Model file for the job. Use its own axes, mm. Coordinates: 2 decimals unless noted, no trailing zeros. Order: outer loops, then holes, each group sorted by start corner. A loop starts at its lowest first (then second) coordinate and runs counter-clockwise, first axis right, second up. Notation, with made-up numbers: M 3.25,44 L 62.25,44 A19 cw 62.25,53 Z; hole C -37.75,-38.75 d6. An arc over 180 degrees is marked long. Return JSON: item names as keys, results as strings.
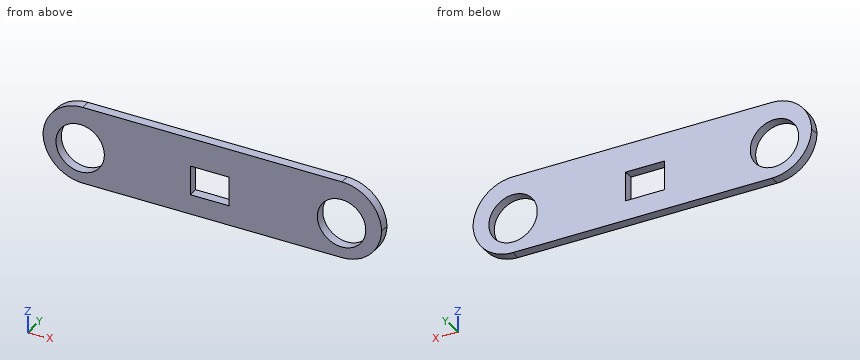
```python
from build123d import *

# Parameters (mm, degrees)
F0_R        = 31.75
F0_W        = 50.8
F0_H        = 38.4544562548
F1_DEPTH    = 12.7
F2_T1_DEPTH = 273.2826573419
F2_T3_DEPTH = 273.264091489
F2_T5_DEPTH = 273.3012245177


# Not quite as in the source:
# - a fillet or chamfer that OpenCascade refuses, or shapes differently, is made with other operations: its cross-section is extruded or revolved along the edge and cut away or added


with BuildPart() as f1:
    # F0 (on Front) → F1 (new body)
    with BuildSketch(Plane.XZ):
        Polygon((248.1590109615, 55.626), (-196.0797500385, 55.626), (-196.0869890385, -45.974), (248.1590109615, -45.974), align=None)
        with Locations((-147.3189890385, 0)):
            Circle(F0_R, mode=Mode.SUBTRACT)
        with Locations((22.6070109615, -0.7874006405)):
            Rectangle(F0_W, F0_H, mode=Mode.SUBTRACT)
        with Locations((195.5810109615, 0)):
            Circle(F0_R, mode=Mode.SUBTRACT)
    extrude(amount=F1_DEPTH)

    # F2: fillet of radius 52.1165314684 on 4 edges, made by hand

    # F2_s2 → F2_t1 (cut)
    with BuildSketch(Plane.XZ.offset(-130.291328671)):
        with BuildLine():
            ThreePointArc((196.0424794931, 55.626), (232.8944323064, 40.3614213448), (248.1590109615, 3.5094685316))
            Line((248.1590109615, 3.5094685316), (248.1590109615, 55.626))
            Line((248.1590109615, 55.626), (196.0424794931, 55.626))
        make_face()
        with BuildLine():
            ThreePointArc((196.0424794931, -45.974), (232.8944323064, -30.7094213448), (248.1590109615, 6.1425314684))
            Line((248.1590109615, 6.1425314684), (248.1590109615, -45.974))
            Line((248.1590109615, -45.974), (196.0424794931, -45.974))
        make_face()
    extrude(amount=F2_T1_DEPTH, mode=Mode.SUBTRACT)

    # F2_s4 → F2_t3 (cut)
    with BuildSketch(Plane.XZ.offset(-130.2820457445)):
        with BuildLine():
            ThreePointArc((-143.9669317407, 55.626), (-180.8175716797, 40.3627341723), (-196.0834630768, 3.5131818345))
            Line((-196.0834630768, 3.5131818345), (-196.0797500385, 55.626))
            Line((-196.0797500385, 55.626), (-143.9669317407, 55.626))
        make_face()
    extrude(amount=F2_T3_DEPTH, mode=Mode.SUBTRACT)

    # F2_s6 → F2_t5 (cut)
    with BuildSketch(Plane.XZ.offset(-130.3006122588)):
        with BuildLine():
            ThreePointArc((-196.083275471, 6.1462447712), (-180.8200097756, -30.7081084706), (-143.9667441349, -45.974))
            Line((-143.9667441349, -45.974), (-196.0869890385, -45.974))
            Line((-196.0869890385, -45.974), (-196.083275471, 6.1462447712))
        make_face()
    extrude(amount=F2_T5_DEPTH, mode=Mode.SUBTRACT)


solid = f1.part
```
Item 1: Saw through at A-A (y = -2.5). Write the cut outline in (x, z), and give its area (3 significant figures).
Check result:
{"outline": "M -196.07,4.83 A52.12 ccw -143.97,-45.97 L 196.04,-45.97 A52.12 ccw 248.14,4.83 A52.12 ccw 196.04,55.63 L -143.97,55.63 A52.12 ccw Z; hole C -147.32,0 d63.5; hole M -2.79,-20.01 L 48.01,-20.01 L 48.01,18.44 L -2.79,18.44 Z; hole C 195.58,0 d63.5", "area": "34,500 mm2"}
Item 2: Wall check: line 1 (Z direction, x = 42, y = -5.5); line 2 (X direction, y = -11.25, z = -21); line 3 (X direction, y = -9.25, z = -3). Give the ranges that are in metal, low to high.
Check result:
{"line 1": "z = -45.97 to -20.01, 18.44 to 55.63", "line 2": "x = -188.46 to -171.13, -123.51 to 171.77, 219.39 to 240.53", "line 3": "x = -195.28 to -178.93, -115.71 to -2.79, 48.01 to 163.97, 227.19 to 247.35"}
Item 3: Saw through at C-C (z = 0). Write the cut outline in (x, y), and give its area (3 significant figures).
Check result:
{"outline": "M -195.72,-12.7 L -179.07,-12.7 L -179.07,0 L -195.72,0 Z; M -115.57,-12.7 L -2.79,-12.7 L -2.79,0 L -115.57,0 Z; M 48.01,-12.7 L 163.83,-12.7 L 163.83,0 L 48.01,0 Z; M 227.33,-12.7 L 247.8,-12.7 L 247.8,0 L 227.33,0 Z", "area": "3,370 mm2"}
Item 4: Drop flat-ended pins along their axis: pin 1 Ø2 at (y, z) = (-8, 22.5) entering from -X; pin 2 Ø2 at (y, z) = (-3.5, 43.5) entering from -X; pin 3 Ø6 at (y, z) = (-3, -23) entering from -X. Give the stop position or say it passes through.
Check result:
{"pin 1": "stops at x = -192.88", "pin 2": "stops at x = -178.55", "pin 3": "stops at x = -189.05"}
Item 5: Saw through at B-B (z = 25). Write the cut outline in (x, y).
Check result:
{"outline": "M -191.45,-12.7 L -166.89,-12.7 L -166.89,0 L -191.45,0 Z; M -127.75,-12.7 L 176.01,-12.7 L 176.01,0 L -127.75,0 Z; M 215.15,-12.7 L 243.52,-12.7 L 243.52,0 L 215.15,0 Z"}
